Can you work these out from the drawing? Everything is in mm from the part's minimum corner. A direction names the side the tool comes from. Give positions to 0.01 mm unless a question says otherwise; leave off trailing zeros. Loops run counter-clockwise (first coordinate to the right, second up) from the corner with the lowest first, then second, coordinate; pieces in that order, holes last. Notation, with made-up numbers: (23, 25.5) - (78, 25.5) arc R21 ccw to (78, 39.5) - close; hole circle Ø10 at (-9.75, -15.5). An arc over 180 degrees is marked (long way). Answer in a Markdown table with one row per item. Add a question column.
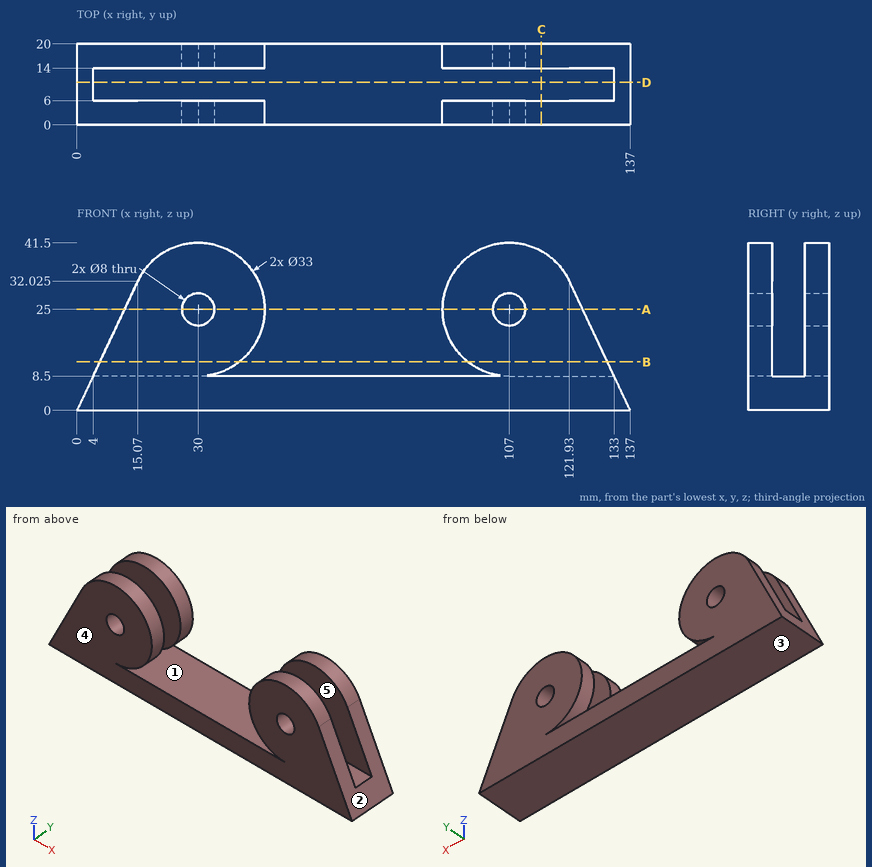
(1) I want a section at A-A on z = 25. State how many separate pieces and enclosed holes the cut face has.
(2) We'd pull the mould along X, two halves only. Please class the marked faces 1, 2 and 3: pulls with the +X half, pulls with the -X half, needs draft (parallel to the pull), parting line crosses it, or undercut.
(3) For pin 1 Ø10 at (x, y) = (92, 7.5) entering from +Z (1 decimal); pin 2 Ø6 at (y, z) = (15.5, 33) entering from -X; pin 3 Ø2 at (x, y) = (49, 11) entering from +Z, each with a flat end and sliding along its axis, tell me the tip position at first contact or that it passes through.
(4) Please list where these lines run through material, in increasing order: line 1 (Y direction, x = 113, z = 32.5); line 2 (X direction, y = 2.7, z = 25) (1 decimal); line 3 (X direction, y = 17.75, z = 26) (1 decimal).
(5) I want a section at C-C on x = 115. Please give me the cut outline in (y, z).
(6) On a 3-axis mill with a long thin cutter (end or side, diameter ignored), from which of +Z, -Z, +X, -X, +Y, -Y can I reach the whole of each face in a straight line? I mean the marked faces 4 and 5. Say none if no direction works.
(7) I want a section at D-D on y = 10.5. Please give me the cut outline in (x, z).
(8) I want a section at B-B on z = 12. Please give me the cut outline in (x, y).
Reported:
| question | item | result |
|---|---|---|
| 1 | separate pieces | 8 |
| 1 | enclosed holes | 0 |
| 2 | face 1 | undercut |
| 2 | face 2 | pulls with the +X half |
| 2 | face 3 | needs draft |
| 3 | pin 1 | z = 37.9 |
| 3 | pin 2 | x = 14.12 |
| 3 | pin 3 | z = 8.5 |
| 4 | line 1 | 0 to 6, 14 to 20 |
| 4 | line 2 | 11.8 to 26, 34 to 46.5, 90.5 to 103, 111 to 125.2 |
| 4 | line 3 | 12.2 to 26.1, 33.9 to 46.5, 90.5 to 103.1, 110.9 to 124.8 |
| 5 | outline | (0, 0) - (20, 0) - (20, 39.43) - (14, 39.43) - (14, 8.5) - (6, 8.5) - (6, 39.43) - (0, 39.43) - close |
| 6 | face 4 | +Z, -Z, +X, -X, -Y |
| 6 | face 5 | +Z, +X, -X |
| 7 | outline | (0, 0) - (137, 0) - (133, 8.5) - (4, 8.5) - close |
| 8 | outline | (5.65, 0) - (40.16, 0) - (40.16, 6) - (5.65, 6) - close; (5.65, 14) - (40.16, 14) - (40.16, 20) - (5.65, 20) - close; (96.84, 0) - (131.35, 0) - (131.35, 6) - (96.84, 6) - close; (96.84, 14) - (131.35, 14) - (131.35, 20) - (96.84, 20) - close |
